Could you check a few things on this model? Use its own coordinates, in mm. A direction names the side the tool comes from. Give positions to 0.01 mm unless a question says otherwise; leave off trailing zeros. Order: outer loops, then holes, each group sorted by start corner. A loop starts at its lowest first (then second) coordinate and runs counter-clockwise, first axis right, second up. Notation, with made-up numbers: (-30.75, 69) - (-24.75, 69) arc R9 cw to (-24.75, 81) - close; hole circle Ø9 at (16, 88). An arc over 180 degrees is marked (long way). Put each result on its own line as item: value.
from build123d import *

# Parameters (mm, degrees)
F0_W     = 39.5
F0_H     = 20
F1_DEPTH = 10
F2_R     = 1.55
F3_DEPTH = 25
F4_W     = 21.086062
F4_H     = 7.881046
F5_DEPTH = 2.5
F7_DEPTH = 6
F8_R     = 3.136424
F9_DEPTH = 7.5


with BuildPart() as f1:
    # F0 (on Front) → F1 (new body)
    with BuildSketch(Plane.XZ):
        with Locations((19.75, 10)):
            Rectangle(F0_W, F0_H)
    extrude(amount=F1_DEPTH)

    # F2 (on face) → F3 (cut)
    with BuildSketch(Plane.XZ.offset(10)):
        with Locations((29.25, 10)):
            Circle(F2_R)
    extrude(amount=-F3_DEPTH, mode=Mode.SUBTRACT)

    # F4 (on face) → F5 (join)
    with BuildSketch(Plane.XZ.offset(10)):
        with Locations((11.988713, 9.816159)):
            Rectangle(F4_W, F4_H)
    extrude(amount=F5_DEPTH)

    # F6 (on face) → F7 (join)
    with BuildSketch(Plane.XZ.offset(12.5)):
        with BuildLine():
            Line((18.691611, 9.816159), (17.741611, 9.816159))
            ThreePointArc((17.741611, 9.816159), (18.691611, 8.866159), (19.641611, 9.816159))
            Line((19.641611, 9.816159), (18.691611, 9.816159))
        make_face()
        with BuildLine():
            ThreePointArc((19.641611, 9.816159), (18.691611, 10.766159), (17.741611, 9.816159))
            Line((17.741611, 9.816159), (18.691611, 9.816159))
            Line((18.691611, 9.816159), (19.641611, 9.816159))
        make_face()
        with BuildLine():
            ThreePointArc((10.141611, 9.816159), (9.191611, 10.766159), (8.241611, 9.816159))
            Line((8.241611, 9.816159), (9.191611, 9.816159))
            Line((9.191611, 9.816159), (10.141611, 9.816159))
        make_face()
        with BuildLine():
            Line((9.191611, 9.816159), (8.241611, 9.816159))
            ThreePointArc((8.241611, 9.816159), (9.191611, 8.866159), (10.141611, 9.816159))
            Line((10.141611, 9.816159), (9.191611, 9.816159))
        make_face()
    extrude(amount=F7_DEPTH)

    # F8 (on face) → F9 (cut)
    with BuildSketch(Plane.XZ.offset(10)):
        with Locations((29.25, 10)):
            Circle(F8_R)
    extrude(amount=-F9_DEPTH, mode=Mode.SUBTRACT)


solid = f1.part
1) I'm going to push flat-ended pins straight in: pin 1 (5 mm diameter, centred on y = -11.5, z = 10.5, fed in from -X); pin 2 (3 mm diameter, centred on y = -16.5, z = 12, fed in from -X); pin 3 (5 mm diameter, centred on x = 30.5, z = 10.5, fed in from -Y); pin 4 (0.8 mm diameter, centred on y = -11, z = 11.5, fed in from -X). Where does each tip first touch, or does it pass through?
Filled in:
pin 1: stops at x = 0
pin 2: stops at x = 8.53
pin 3: stops at y = -10
pin 4: stops at x = 1.45
2) Suppose I cut it at C-C, the plane x = 14.5. List the corners of the cut face in (y, z) for me, and give its area (3 significant figures).
Filled in:
outline: (-12.5, 5.88) - (-10, 5.88) - (-10, 0) - (0, 0) - (0, 20) - (-10, 20) - (-10, 13.76) - (-12.5, 13.76) - close
area: 220 mm^2
3) Suppose I cut it at D-D, the plane z = 18.5. List the corners of the cut face in (x, y) for me.
Filled in:
outline: (0, -10) - (39.5, -10) - (39.5, 0) - (0, 0) - close
4) Suppose I cut it at B-B, the plane y = -4.25. List the corners of the cut face in (x, z) for me, and give its area (3 significant figures).
Filled in:
outline: (0, 0) - (39.5, 0) - (39.5, 20) - (0, 20) - close; hole circle Ø6.27 at (29.25, 10)
area: 759 mm^2
5) Which directions (+Z, -Z, +X, -X, +Y, -Y) give clear straight access to the entire face, cutting with the end or side of a thin tool? Please do faces 1 (the flat face through (12, -11, 5.876)), 2 (the cylindrical face through (17.938, -15.458, 9.238)), 3 (the flat face through (19, -18.5, 10)).
Filled in:
face 1: -Z, +X, -X, -Y
face 2: -Y
face 3: +Z, -Z, +X, -X, -Y
6) We'd pull the mould along X, two halves only. Please class faces 4 (the flat face through (1.446, -11, 10)), 5 (the flat face through (22.532, -11, 10)), 6 (the flat face through (12, -11, 13.757)), 7 (the flat face through (31, -2.5, 9)): pulls with the +X half, pulls with the -X half, needs draft (parallel to the pull), parting line crosses it, or undercut.
Filled in:
face 4: pulls with the -X half
face 5: pulls with the +X half
face 6: needs draft
face 7: undercut
7) Suppose I cut it at A-A, the plane x = 29.25. List the corners of the cut face in (y, z) for me.
Filled in:
outline: (-10, 0) - (0, 0) - (0, 8.45) - (-2.5, 8.45) - (-2.5, 6.86) - (-10, 6.86) - close; (-10, 13.14) - (-2.5, 13.14) - (-2.5, 11.55) - (0, 11.55) - (0, 20) - (-10, 20) - close
8) If I drill on line 1 (Z direction, x = 29.25, y = -6); line 2 (Y direction, x = 33, z = 4); line 3 (Y direction, x = 15, z = 7), over which ranges is the centre line in solid material (lowest first)? Write a range as [from, to].
Filled in:
line 1: z = [0, 6.86], [13.14, 20]
line 2: y = [-10, 0]
line 3: y = [-12.5, 0]
